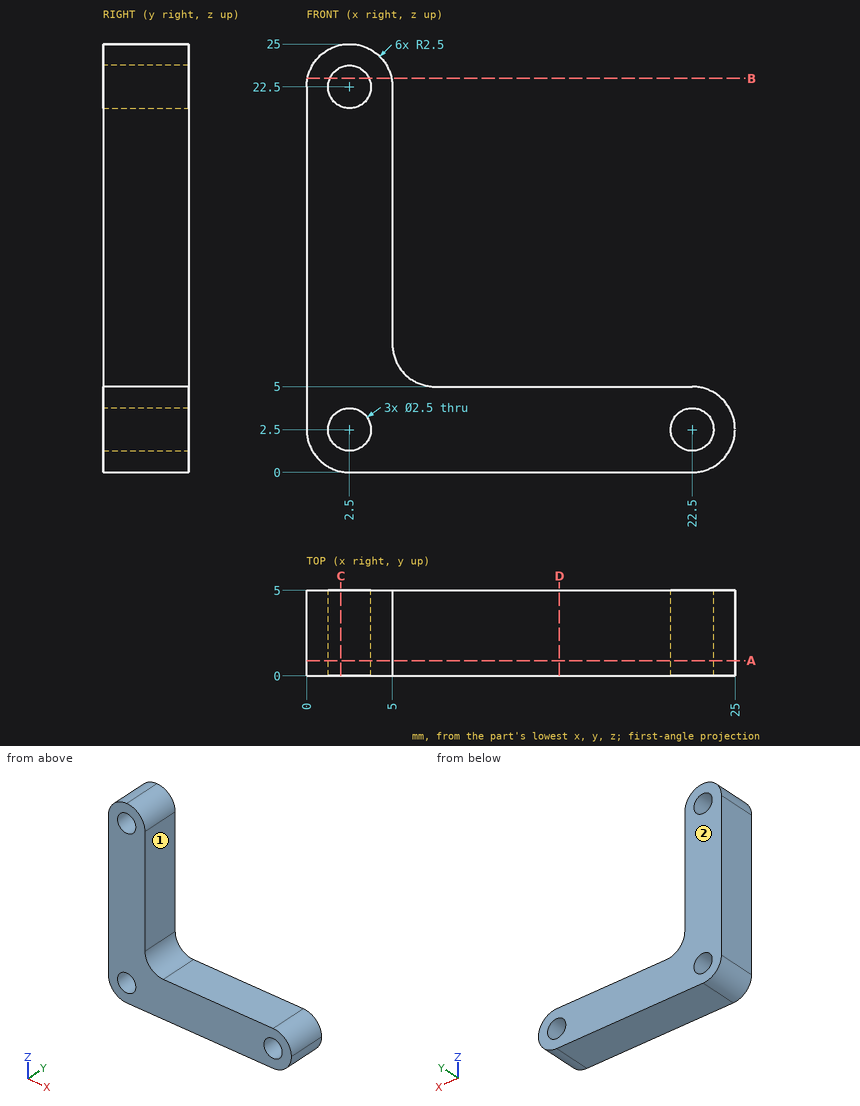
Print and shaded views of the part. All mm, measured from the part's lowest x, y and z. A direction names the side the tool comes from. Round coordinates to 2 decimals unless told otherwise and drop trailing zeros. Order: outer loops, then holes, each group sorted by start corner. A loop starts at its lowest first (then second) coordinate and runs counter-clockwise, first axis right, second up.
Q1. Slice it at B-B (z = 23). Write the cut outline in (x, y), and give its area (3 significant figures).
Q2. Drop flat-ended pins along their axis: pin 1 (3 mm diameter, centred on x = 17.5, y = 1, fed in from +Z); pin 2 (1.5 mm diameter, centred on y = 3, z = 15.5, fed in from +X); pin 3 (2 mm diameter, centred on x = 22.5, z = 2.5, fed in from -Y). Give the stop position or say it passes through.
Q3. Slice it at C-C (x = 2). Write the cut outline in (y, z), and give its area (3 significant figures).
Q4. Slice it at D-D (x = 14.75). Write the cut outline in (y, z).
Q5. Which spindle directions (+Z, -Z, +X, -X, +Y, -Y) get a long thin tool onto all of the face, cutting with end or side? Do the marked faces 1 and 2. Say none if no direction does.
Q6. Slice it at A-A (y = 0.9). State how many separate pieces and enclosed holes the cut face has, and give its area (3 significant figures).
Q7. Wall check: L1, parallel to X at y = 3.2, z = 2.5; L2, parallel to X at y = 2.35, z = 22.5; L3, parallel to X at y = 1.95, z = 3.5. Give the ranges that are in metal, low to high.
Results below:
1. outline: (0.05, 0) - (1.35, 0) - (1.35, 5) - (0.05, 5) - close; (3.65, 0) - (4.95, 0) - (4.95, 5) - (3.65, 5) - close
1. area: 13.0 mm2
2. pin 1: stops at z = 5
2. pin 2: stops at x = 5
2. pin 3: passes through
3. outline: (0, 0.05) - (5, 0.05) - (5, 1.35) - (0, 1.35) - close; (0, 3.65) - (5, 3.65) - (5, 21.35) - (0, 21.35) - close; (0, 23.65) - (5, 23.65) - (5, 24.95) - (0, 24.95) - close
3. area: 102 mm2
4. outline: (0, 0) - (5, 0) - (5, 5) - (0, 5) - close
5. face 1: +Z, +X, +Y, -Y
5. face 2: +Z, -Z, +X, -X, +Y
6. separate pieces: 1
6. enclosed holes: 3
6. area: 205 mm2
7. L1: x = 0 to 1.25, 3.75 to 21.25, 23.75 to 25
7. L2: x = 0 to 1.25, 3.75 to 5
7. L3: x = 0 to 1.75, 3.25 to 21.75, 23.25 to 24.79
